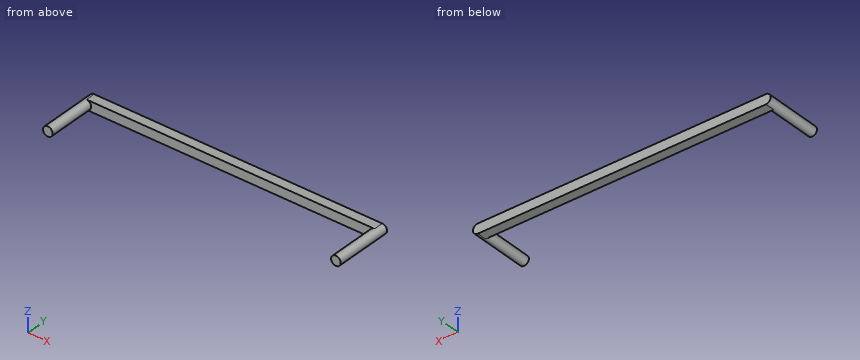
from build123d import *
from build123d.topology import SkipClean

# Parameters (mm, degrees)
SALIENTE_EXTRUIR1_DEPTH = 2
SALIENTE_EXTRUIR2_START = -12
CROQUIS2_R              = 1
SALIENTE_EXTRUIR2_DEPTH = 12


with BuildPart() as part:
    # Croquis1 → Saliente-Extruir1 (new body)
    with BuildSketch(Plane(origin=(0, -13.655018192, 0), x_dir=(1, 0, 0), z_dir=(0, 1, 0))):
        with BuildLine():
            Line((-15.39391873, -33.464706181), (44.60608127, -33.464706181))
            ThreePointArc((44.60608127, -33.464706181), (45.60608127, -34.464706181), (44.60608127, -35.464706181))
            Line((44.60608127, -35.464706181), (-15.39391873, -35.464706181))
            ThreePointArc((-15.39391873, -35.464706181), (-16.39391873, -34.464706181), (-15.39391873, -33.464706181))
        make_face()
    extrude(amount=SALIENTE_EXTRUIR1_DEPTH)

    # Croquis2 → Saliente-Extruir2 (add)
    with SkipClean():  # the faces are left unmerged after this step: merging them gives an invalid solid
        with BuildSketch(Plane(origin=(0, -11.655018192, 0), x_dir=(1, 0, 0), z_dir=(0, 1, 0)).offset(SALIENTE_EXTRUIR2_START)):
            with Locations(Location((-15.39391873, -34.464706181, 0), (0, 0, 270))):
                Circle(CROQUIS2_R)
            with Locations(Location((44.60608127, -34.464706181, 0), (0, 0, 270))):
                Circle(CROQUIS2_R)
        extrude(amount=SALIENTE_EXTRUIR2_DEPTH)


solid = part.part
Can you work these out from the model? Positions are in its coordinate system, mm. Give positions to 0.01 mm unless a question says otherwise; leave off trailing zeros. Write each loop counter-clockwise with the first axis right and the second up, starting at its lowest first coordinate (ties: lowest second). Pieces come first, ordered by that corner, then holes. Notation, with made-up numbers: M 67.5,-2 L 84.5,-2 A23 ccw 84.5,19 Z; hole C 52.25,26 d8. An arc over 180 degrees is marked long. Answer in a Markdown table with one row per item. Add a question column.
Item 1: Imagine slicing it at C-C, the plane x = 22. Write out the boundary of the cut face in (y, z), plus the area to 3 significant figures.
Item 2: Imagine slicing it at A-A, the plane z = 34.5. Write out the boundary of the cut face in (x, y), plus the area to 3 significant figures.
Item 3: For pin 1 Ø1 at (x, z) = (2.5, 34.5) entering from -Y (3 decimals); pin 2 Ø1 at (x, y) = (18.5, -15.5) entering from -Z, each with a flat end and sliding along its axis, tell me the tip position at first contact or that it passes through.
Item 4: Please list where these lines run through material, in increasing order: L1, parallel to Y at x = 21, z = 34.3; L2, parallel to X at y = -13.75, z = 34.1; L3, parallel to X at y = -19, z = 35.3.
Item 5: Imagine slicing it at B-B, the plane y = -16.25. Write out the boundary of the cut face in (x, z).
Evaluation:
| question | item | result |
|---|---|---|
| 1 | outline | M -13.66,33.46 L -11.66,33.46 L -11.66,35.46 L -13.66,35.46 Z |
| 1 | area | 4.00 mm² |
| 2 | outline | M -16.39,-23.66 L -14.39,-23.66 L -14.39,-13.66 L 43.61,-13.66 L 43.61,-23.66 L 45.61,-23.66 L 45.61,-11.66 L -16.39,-11.66 Z |
| 2 | area | 164 mm² |
| 3 | pin 1 | stops at y = -13.655 |
| 3 | pin 2 | passes through |
| 4 | L1 | y = -13.66 to -11.66 |
| 4 | L2 | x = -16.33 to -14.46, 43.67 to 45.54 |
| 4 | L3 | x = -15.94 to -14.84, 44.06 to 45.16 |
| 5 | outline | C -15.39,34.46 d2; C 44.61,34.46 d2 |
